Read the model definition and answer for the solid it produces. Units are mm, in the model's axes. A direction names the side the tool comes from. Give positions to 0.01 mm unless a question says otherwise; leave off trailing zeros. Loops run counter-clockwise (first coordinate to the right, second up) from the corner with the lowest first, then second, coordinate; pieces in that order, holes last. Notation, with made-up numbers: (58.25, 18.5) -> (92.25, 18.5) arc R24 cw to (92.25, 30.5) -> close; hole circle Ø1 at (60, 34.5). An arc over 180 degrees is marked (long way). Write each question's results on one line, items separated by ' | '. Start each with the question number.
Item 1: Section D-D on x = -319.5 is taken. Write down the section's boundary in (y, z).
Item 2: Find the intervals of material crossed by line 1 (X direction, y = 47.5, z = 13.5); line 2 (X direction, y = 96, z = 13); line 3 (Y direction, x = -330.5, z = 10.5), in increasing order.
Item 3: Each of these flat-tipped pins is pushed along its axis until it touches: P1, Ø2, axis at x = -288.5, z = 21.5, coming from the +Y side; P2, Ø5, axis at x = -475.5, z = 8.5, coming from the -Y side. Where does it stop, or does it pass through?
Item 4: Section C-C on y = 171 is taken. Write down the section's boundary in (x, z).
Item 5: Section A-A on y = 66 is taken. Write down the section's boundary in (x, z).
Item 6: Which of the six approach directions +Z, -Z, +X, -X, +Y, -Y give full straight-line access (tool end or side, diameter ignored) to faces 1 (the flat face through (-267.123, 42, 17)), 2 (the flat face through (-120.91, 438.322, 17.255))?
Item 7: Section B-B on z = 24 is taken. Write down the section's boundary in (x, y), and give its area (3 significant figures).
```python
from build123d import *

# Parameters (mm, degrees)
AUFSATZ_LINEAR_AUSTRAGEN1_DEPTH = 35


with BuildPart() as part:
    # Skizze1 → Aufsatz-Linear austragen1 (new body)
    with BuildSketch(Plane.XY):
        with BuildLine():
            Line((62.877451446, 389.076644167), (62.877451446, 7.806644167))
            Line((62.877451446, 7.806644167), (-267.122548554, 7.806644167))
            Line((-267.122548554, 7.806644167), (-267.122548554, 77.806644167))
            ThreePointArc((-267.122548554, 77.806644167), (-377.122548554, 187.806644167), (-487.122548554, 77.806644167))
            Line((-487.122548554, 77.806644167), (-487.122548554, 7.806644167))
            Line((-487.122548554, 7.806644167), (-817.122548554, 7.806644167))
            Line((-817.122548554, 7.806644167), (-817.122548554, 389.076644167))
            Line((-817.122548554, 389.076644167), (-454.622548554, 486.208226423))
            Line((-454.622548554, 486.208226423), (-299.622548554, 486.208226423))
            Line((-299.622548554, 486.208226423), (62.877451446, 389.076644167))
        make_face()
    extrude(amount=AUFSATZ_LINEAR_AUSTRAGEN1_DEPTH)


solid = part.part
```
Findings:
1) outline: (171.51, 0) -> (486.21, 0) -> (486.21, 35) -> (171.51, 35) -> close
2) line 1: -817.12 to -487.12, -267.12 to 62.88 | line 2: -817.12 to -485.61, -268.64 to 62.88 | line 3: 177.44 to 486.21
3) P1: y = 483.5 | P2: y = 121.67
4) outline: (-817.12, 0) -> (-435.56, 0) -> (-435.56, 35) -> (-817.12, 35) -> close; (-318.68, 0) -> (62.88, 0) -> (62.88, 35) -> (-318.68, 35) -> close
5) outline: (-817.12, 0) -> (-487.12, 0) -> (-487.12, 35) -> (-817.12, 35) -> close; (-267.12, 0) -> (62.88, 0) -> (62.88, 35) -> (-267.12, 35) -> close
6) face 1: +Z, -Z, -Y | face 2: +Z, -Z, +X, +Y
7) outline: (-817.12, 7.81) -> (-487.12, 7.81) -> (-487.12, 77.81) arc R110 cw to (-267.12, 77.81) -> (-267.12, 7.81) -> (62.88, 7.81) -> (62.88, 389.08) -> (-299.62, 486.21) -> (-454.62, 486.21) -> (-817.12, 389.08) -> close | area: 351,000 mm2
